Geometry check sheet. Reference: drawing and pictorial views, mm from the part's lowest x, y, z. A direction names the side the tool comes from. Give positions to 0.01 mm unless a question says otherwise; leave off trailing zeros. Write each loop counter-clockwise with the first axis right and the second up, starting at its lowest first coordinate (ties: lowest second). Pieces come first, ordered by that corner, then holes. Notation, with made-up numbers: (-14, 61.5) -> (13, 61.5) arc R28 ccw to (13, 85.5) -> close; hole circle Ø1 at (26.25, -28.5). An arc over 180 degrees is marked (long way). Return JSON: item names as keys, results as strings.
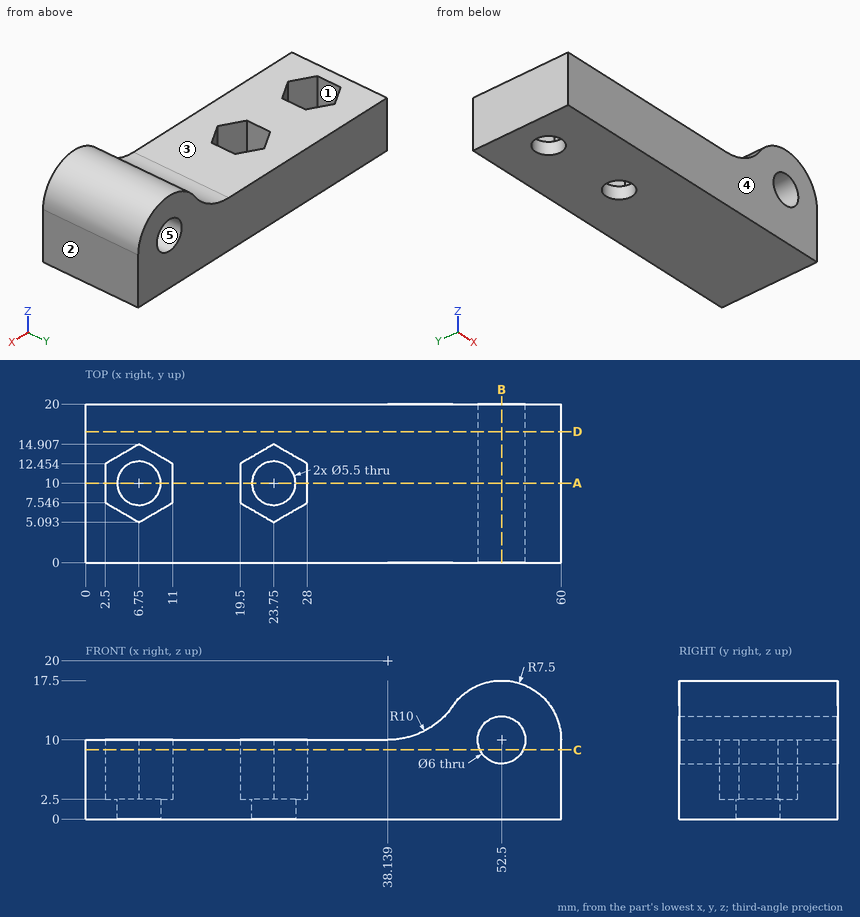
(1) Cross-section at C-C on z = 8.75. Enter the section's corners in (x, y).
Reply:
{"outline": "(0, 0) -> (49.77, 0) -> (49.77, 20) -> (0, 20) -> close; (55.23, 0) -> (60, 0) -> (60, 20) -> (55.23, 20) -> close; hole (2.5, 7.55) -> (6.75, 5.09) -> (11, 7.55) -> (11, 12.45) -> (6.75, 14.91) -> (2.5, 12.45) -> close; hole (19.5, 7.55) -> (23.75, 5.09) -> (28, 7.55) -> (28, 12.45) -> (23.75, 14.91) -> (19.5, 12.45) -> close"}
(2) Set-up check for the marked faces 1 and 2: record each of +Z, -Z, +X, -X, +Y, -Y from which the full face is reachable in a straight line by a thin tool's end or side.
Reply:
{"face 1": "+Z", "face 2": "+Z, -Z, +X, +Y, -Y"}
(3) Thickness scan on L1, parallel to X at y = 8.25, z = 3.5; L2, parallel to Y at x = 6.75, z = 2.05; L3, parallel to Z at x = 52.5, y = 13.25. Record the ranges inside material, lowest first.
Reply:
{"L1": "0 to 2.5, 11 to 19.5, 28 to 60", "L2": "0 to 7.25, 12.75 to 20", "L3": "0 to 7, 13 to 17.5"}
(4) Release check for a two-part mould opening along Z. For the marked faces 3, 4 and 5 record: pulls with the +Z half, pulls with the -Z half, needs draft (parallel to the pull), parting line crosses it, or undercut.
Reply:
{"face 3": "pulls with the +Z half", "face 4": "needs draft", "face 5": "undercut"}
(5) Depth check by flat-ended pin: pin 1 Ø3 at (x, y) = (32.5, 18) entering from +Z; pin 2 Ø7 at (x, y) = (23.75, 10) entering from +Z. Enter the tip coordinate at first touch or a pass-through.
Reply:
{"pin 1": "z = 10", "pin 2": "z = 2.5"}
(6) Cross-section at D-D on y = 16.5. Enter the section's corners in (x, z) (1 decimal).
Reply:
{"outline": "(0, 0) -> (60, 0) -> (60, 10) arc R7.5 ccw to (46.3, 14.3) arc R10 cw to (38.1, 10) -> (0, 10) -> close; hole circle Ø6 at (52.5, 10)"}
(7) Cross-section at B-B on x = 52.5. Enter the section's corners in (y, z).
Reply:
{"outline": "(0, 0) -> (20, 0) -> (20, 7) -> (0, 7) -> close; (0, 13) -> (20, 13) -> (20, 17.5) -> (0, 17.5) -> close"}
(8) Cross-section at A-A on y = 10. Enter the section's corners in (x, z) (1 decimal).
Reply:
{"outline": "(0, 0) -> (4, 0) -> (4, 2.5) -> (2.5, 2.5) -> (2.5, 10) -> (0, 10) -> close; (9.5, 0) -> (21, 0) -> (21, 2.5) -> (19.5, 2.5) -> (19.5, 10) -> (11, 10) -> (11, 2.5) -> (9.5, 2.5) -> close; (26.5, 0) -> (60, 0) -> (60, 10) arc R7.5 ccw to (46.3, 14.3) arc R10 cw to (38.1, 10) -> (28, 10) -> (28, 2.5) -> (26.5, 2.5) -> close; hole circle Ø6 at (52.5, 10)"}
